Verification items for the finished model (mm, model axes). Give positions to 0.01 mm unless a question says otherwise; leave off trailing zeros. Answer as a JSON object with one key per item and string values.
```python
from build123d import *

# Parameters (mm, degrees)
ESTRUSIONE_ESTRUSIONE1_DEPTH = 500
SCHIZZO2_R                   = 4.005
ESTRUSIONE_ESTRUSIONE4_DEPTH = 20
SCHIZZO6_R                   = 4
TAGLIO_ESTRUSIONE20_DEPTH    = 20


with BuildPart() as part:
    # Schizzo1 → Estrusione-Estrusione1 (new body)
    with BuildSketch(Plane.XY):
        with BuildLine():
            Line((-4, -3), (-4, 3))
            Line((-4, 3), (-7, 6))
            Line((-7, 6), (-8, 6))
            Line((-8, 6), (-8, 3))
            Line((-8, 3), (-9.5, 3))
            ThreePointArc((-9.5, 3), (-9.853553391, 3.146446609), (-10, 3.5))
            Line((-10, 3.5), (-10, 9))
            ThreePointArc((-10, 9), (-9.707106781, 9.707106781), (-9, 10))
            Line((-9, 10), (-3.5, 10))
            ThreePointArc((-3.5, 10), (-3.146446609, 9.853553391), (-3, 9.5))
            Line((-3, 9.5), (-3, 8))
            Line((-3, 8), (-6, 8))
            Line((-6, 8), (-6, 7))
            Line((-6, 7), (-3, 4))
            Line((-3, 4), (3, 4))
            Line((3, 4), (6, 7))
            Line((6, 7), (6, 8))
            Line((6, 8), (3, 8))
            Line((3, 8), (3, 9.5))
            ThreePointArc((3, 9.5), (3.146446609, 9.853553391), (3.5, 10))
            Line((3.5, 10), (9, 10))
            ThreePointArc((9, 10), (9.707106781, 9.707106781), (10, 9))
            Line((10, 9), (10, 3.5))
            ThreePointArc((10, 3.5), (9.853553391, 3.146446609), (9.5, 3))
            Line((9.5, 3), (8, 3))
            Line((8, 3), (8, 6))
            Line((8, 6), (7, 6))
            Line((7, 6), (4, 3))
            Line((4, 3), (4, -3))
            Line((4, -3), (7, -6))
            Line((7, -6), (8, -6))
            Line((8, -6), (8, -3))
            Line((8, -3), (9.5, -3))
            ThreePointArc((9.5, -3), (9.853553391, -3.146446609), (10, -3.5))
            Line((10, -3.5), (10, -9))
            ThreePointArc((10, -9), (9.707106781, -9.707106781), (9, -10))
            Line((9, -10), (3.5, -10))
            ThreePointArc((3.5, -10), (3.146446609, -9.853553391), (3, -9.5))
            Line((3, -9.5), (3, -8))
            Line((3, -8), (6, -8))
            Line((6, -8), (6, -7))
            Line((6, -7), (3, -4))
            Line((3, -4), (-3, -4))
            Line((-3, -4), (-6, -7))
            Line((-6, -7), (-6, -8))
            Line((-6, -8), (-3, -8))
            Line((-3, -8), (-3, -9.5))
            ThreePointArc((-3, -9.5), (-3.146446609, -9.853553391), (-3.5, -10))
            Line((-3.5, -10), (-9, -10))
            ThreePointArc((-9, -10), (-9.707106781, -9.707106781), (-10, -9))
            Line((-10, -9), (-10, -3.5))
            ThreePointArc((-10, -3.5), (-9.853553391, -3.146446609), (-9.5, -3))
            Line((-9.5, -3), (-8, -3))
            Line((-8, -3), (-8, -6))
            Line((-8, -6), (-7, -6))
            Line((-7, -6), (-4, -3))
        make_face()
    extrude(amount=ESTRUSIONE_ESTRUSIONE1_DEPTH)

    # Schizzo2 → Estrusione-Estrusione4 (add)
    with BuildSketch(Plane.ZY.offset(10)):
        with Locations((25, 0)):
            Circle(SCHIZZO2_R)
        with Locations((475, 0)):
            Circle(SCHIZZO2_R)
    extrude(amount=-ESTRUSIONE_ESTRUSIONE4_DEPTH)

    # Schizzo6 → Taglio-Estrusione20 (cut)
    with BuildSketch(Plane.ZY.offset(10)):
        with Locations((25, 0)):
            Circle(SCHIZZO6_R)
        with Locations((475, 0)):
            Circle(SCHIZZO6_R)
    extrude(amount=-TAGLIO_ESTRUSIONE20_DEPTH, mode=Mode.SUBTRACT)


solid = part.part
```
(1) Release check for a two-part mould opening along Z. For faces 1 (the cylindrical face through (-0.1, -2.4, 21.8)), 2 (the flat face through (10, 4, 246)), 3 (the flat face through (0, 0, 0)), 4 (the flat face through (0, 0, 500)) record: pulls with the +Z half, pulls with the -Z half, needs draft (parallel to the pull), parting line crosses it, or undercut.
Computed values:
{"face 1": "undercut", "face 2": "needs draft", "face 3": "pulls with the -Z half", "face 4": "pulls with the +Z half"}
(2) Material ranges on line 1 along Z through (x, y) = (1, -3.5); line 2 along X through (y, z) = (-7.5, 451.5); line 3 along X through (y, z) = (8.5, 213.5), recorded low to high. Write a range as [from, to].
Computed values:
{"line 1": "z = [0, 23.06], [26.94, 473.06], [476.94, 500]", "line 2": "x = [-10, -6], [6, 10]", "line 3": "x = [-10, -3], [3, 10]"}
(3) Gauge pin test, flat end, axial feed: pin 1 Ø1.8 at (x, z) = (-0.5, 491) entering from -Y. Record the tip position at first contact, or that the pin passes through.
Computed values:
{"pin 1": "stops at y = -4"}
